Source: CAD feature listing. Evaluate the final solid. Frame: model axes, mm. A direction names the side the tool comes from. Give positions to 0.01 mm unless a question says otherwise; leave off trailing zeros. Loops run counter-clockwise (first coordinate to the right, second up) from the corner with the lowest first, then second, coordinate; pieces in that order, holes last. Notation, with made-up numbers: (37, 87.25) - (65, 87.25) arc R33 cw to (65, 124.25) - close; hole circle Ø3 at (20, 4.25). An arc over 180 degrees is marked (long way). Put each result on its own line as item: value.
```python
from build123d import *

# Parameters (mm, degrees)
SKETCH1_R           = 2
BOSS_EXTRUDE1_DEPTH = 1.6
SKETCH1_3_W         = 8.2
SKETCH1_3_H         = 8.2
SKETCH1_3_W_2       = 6.2
SKETCH1_3_H_2       = 6.2
BOSS_EXTRUDE2_DEPTH = 2
BOSS_EXTRUDE3_START = -0.5
SKETCH1_4_W         = 8.2
SKETCH1_4_H         = 8.2
SKETCH1_4_W_2       = 6.2
SKETCH1_4_H_2       = 6.2
SKETCH1_4_R         = 2
BOSS_EXTRUDE3_DEPTH = 0.5
SKETCH3_W           = 5.8
SKETCH3_H           = 5.8
BOSS_EXTRUDE4_DEPTH = 4.5
CHAMFER1_SIZE       = 0.5
CUT_EXTRUDE1_DEPTH  = 0.2


with BuildPart() as part:
    # Sketch1 → Boss-Extrude1 (new body)
    with BuildSketch(Plane(origin=(0, 0, 0), x_dir=(1, 0, 0), z_dir=(0, 1, 0))):
        with Locations(Location((0, 0, 0), (0, 0, 270))):
            Circle(SKETCH1_R)
    extrude(amount=BOSS_EXTRUDE1_DEPTH)



with BuildPart() as body_2:
    # Sketch1_3 → Boss-Extrude2 (new body)
    with BuildSketch(Plane(origin=(0, 0, 0), x_dir=(1, 0, 0), z_dir=(0, 1, 0))):
        Rectangle(SKETCH1_3_W, SKETCH1_3_H)
        Rectangle(SKETCH1_3_W_2, SKETCH1_3_H_2, mode=Mode.SUBTRACT)
    extrude(amount=BOSS_EXTRUDE2_DEPTH)


with BuildPart() as part_1:
    add(part.part)

    add(body_2.part)  # Boss-Extrude3 merges body 2
    # Sketch1_4 → Boss-Extrude3 (add)
    # profile 1 of 3: a face of its own
    with BuildSketch(Plane(origin=(0, 0, 0), x_dir=(1, 0, 0), z_dir=(0, 1, 0)).offset(BOSS_EXTRUDE3_START)):
        Rectangle(SKETCH1_4_W, SKETCH1_4_H)
        Rectangle(SKETCH1_4_W_2, SKETCH1_4_H_2, mode=Mode.SUBTRACT)
    # profile 2 of 3: a face of its own
    with BuildSketch(Plane(origin=(0, 0, 0), x_dir=(1, 0, 0), z_dir=(0, 1, 0)).offset(BOSS_EXTRUDE3_START)):
        Rectangle(SKETCH1_4_W_2, SKETCH1_4_H_2)
        with Locations(Location((0, 0, 0), (0, 0, 270))):
            Circle(SKETCH1_4_R, mode=Mode.SUBTRACT)
    # profile 3 of 3: a face of its own
    with BuildSketch(Plane(origin=(0, 0, 0), x_dir=(1, 0, 0), z_dir=(0, 1, 0)).offset(BOSS_EXTRUDE3_START)):
        with Locations(Location((0, 0, 0), (0, 0, 270))):
            Circle(SKETCH1_4_R)
    extrude(amount=BOSS_EXTRUDE3_DEPTH)

    # Sketch3 → Boss-Extrude4 (add)
    with BuildSketch(Plane.XZ.offset(0.5)):
        Rectangle(SKETCH3_W, SKETCH3_H)
    extrude(amount=BOSS_EXTRUDE4_DEPTH)

    # Chamfer1
    chamfer1_edges = [part_1.edges().sort_by_distance(p)[0] for p in [
        (2.9, -2.75, -2.9),
        (2.9, -2.75, 2.9),
        (-2.9, -2.75, 2.9),
        (-2.9, -2.75, -2.9),
        (-4.1, 0.75, -4.1),
        (4.1, 0.75, -4.1),
        (4.1, 0.75, 4.1),
        (-4.1, 0.75, 4.1),
    ]]
    chamfer(chamfer1_edges, length=CHAMFER1_SIZE)

    # Sketch4 → Cut-Extrude1 (cut)
    with BuildSketch(Plane.XZ.offset(5)):
        with BuildLine():
            Line((-0.810649843, 2.028880102), (-0.127757215, 2.028880102))
            add(Edge.make_bspline(
                [(-0.127757215, 2.028880102), (-0.094328737, 2.028704351), (-0.029536026, 2.028363703), (0.064683416, 2.023080572), (0.152932226, 2.015876902), (0.235235999, 2.00444681), (0.311556701, 1.990655032), (0.382124338, 1.973953216), (0.44671451, 1.953926603), (0.523827247, 1.922080321), (0.611747908, 1.874757153), (0.7069463, 1.804828588), (0.78835054, 1.719296125), (0.858536857, 1.622813469), (0.914337977, 1.516677698), (0.954707274, 1.403418509), (0.980265149, 1.284496767), (0.982893584, 1.202853589), (0.984221952, 1.161592441)],
                knots=[0, 0, 0, 0, 1.001505555, 1.941167018, 2.826882275, 3.653841531, 4.429895133, 5.150066043, 5.825578002, 6.45369114, 7.647487171, 8.808567382, 9.977351308, 11.170798116, 12.373658725, 13.556498008, 14.765093433, 16, 16, 16, 16], degree=3))
            add(Edge.make_bspline(
                [(0.984221952, 1.161592441), (0.983128733, 1.122939886), (0.980980456, 1.046983969), (0.960437697, 0.935889859), (0.928277028, 0.830138641), (0.883571779, 0.730116255), (0.825469783, 0.638082642), (0.756611464, 0.553295376), (0.673534662, 0.479344319), (0.611291422, 0.438001416), (0.579674676, 0.417001095)],
                knots=[0, 0, 0, 0, 1.044552857, 2.05264487, 3.044412934, 4.028983338, 5.005914585, 5.980388656, 6.974128949, 8, 8, 8, 8], degree=3))
            add(Edge.make_bspline(
                [(0.579674676, 0.417001095), (0.619435104, 0.401736096), (0.695506651, 0.372530372), (0.800192664, 0.320894908), (0.890387509, 0.264732798), (0.966784655, 0.203400947), (1.03212231, 0.137292137), (1.089175251, 0.065437022), (1.137856625, -0.013101736), (1.179569549, -0.097505271), (1.212118305, -0.186911739), (1.236494209, -0.280482515), (1.250461658, -0.377882071), (1.2524493, -0.44416745), (1.253452721, -0.477630315)],
                knots=[0, 0, 0, 0, 1.27268992, 2.434971085, 3.483601985, 4.442670788, 5.356604649, 6.2567628, 7.179492994, 8.113709626, 9.066344395, 10.018646069, 10.999752585, 12, 12, 12, 12], degree=3))
            add(Edge.make_bspline(
                [(1.253452721, -0.477630315), (1.252475875, -0.511797187), (1.250553903, -0.579021465), (1.236373931, -0.6777766), (1.212364824, -0.772151546), (1.179293678, -0.862756729), (1.136131363, -0.949416864), (1.083603399, -1.032230128), (1.020971835, -1.110364458), (0.950908966, -1.184688081), (0.871646821, -1.251515869), (0.786131066, -1.311031575), (0.693284746, -1.359977637), (0.594632752, -1.401093659), (0.489068436, -1.432500857), (0.377065829, -1.454473431), (0.258721527, -1.469278468), (0.177511776, -1.470495673), (0.13586458, -1.471119898)],
                knots=[0, 0, 0, 0, 0.978564426, 1.925352924, 2.850884081, 3.763762016, 4.682927383, 5.618979971, 6.567305752, 7.547517671, 8.540179244, 9.531824382, 10.526200242, 11.540722885, 12.589160233, 13.674978461, 14.80764778, 16, 16, 16, 16], degree=3))
            Line((0.13586458, -1.471119898), (-0.810649843, -1.471119898))
            Line((-0.810649843, -1.471119898), (-0.810649843, 2.028880102))
        make_face()
        with BuildLine():
            Line((-0.496547279, 1.669905743), (-0.496547279, 0.548110871))
            Line((-0.496547279, 0.548110871), (-0.285509619, 0.548110871))
            add(Edge.make_bspline(
                [(-0.285509619, 0.548110871), (-0.254660823, 0.548510794), (-0.195054664, 0.549283527), (-0.108734767, 0.551497044), (-0.028609749, 0.557695087), (0.045182084, 0.563891349), (0.112524528, 0.573965937), (0.173268389, 0.58595806), (0.228366986, 0.598640965), (0.291906532, 0.620210452), (0.36397948, 0.652088127), (0.440812584, 0.701559963), (0.508547054, 0.760484316), (0.565744242, 0.828475278), (0.612555712, 0.903341464), (0.645069427, 0.983888344), (0.667116712, 1.068108476), (0.669108243, 1.125926729), (0.670119388, 1.155282345)],
                knots=[0, 0, 0, 0, 1.156816544, 2.235205308, 3.236616184, 4.169592532, 5.011045266, 5.787822928, 6.49130361, 7.128639758, 8.301311294, 9.436451833, 10.541879658, 11.654887649, 12.756523258, 13.837046038, 14.901820046, 16, 16, 16, 16], degree=3))
            add(Edge.make_bspline(
                [(0.670119388, 1.155282345), (0.669593208, 1.174708117), (0.668561048, 1.212813889), (0.660107745, 1.268363243), (0.645740171, 1.320606996), (0.627285877, 1.370261106), (0.601497189, 1.415772956), (0.571133725, 1.458716152), (0.534448035, 1.49762827), (0.492690722, 1.533997769), (0.4446821, 1.566242296), (0.390450808, 1.59448306), (0.329263131, 1.617223836), (0.262150276, 1.637139989), (0.188079188, 1.651128283), (0.107904635, 1.66278167), (0.020969916, 1.668714412), (-0.039175187, 1.669499775), (-0.070265228, 1.669905743)],
                knots=[0, 0, 0, 0, 0.91205012, 1.789085906, 2.630437955, 3.453916878, 4.269457761, 5.079663411, 5.91843418, 6.774407191, 7.675494373, 8.627863946, 9.638891023, 10.736472738, 11.911756761, 13.175263542, 14.539845004, 16, 16, 16, 16], degree=3))
            Line((-0.070265228, 1.669905743), (-0.496547279, 1.669905743))
        make_face(mode=Mode.SUBTRACT)
        with BuildLine():
            Line((-0.496547279, 0.189136512), (-0.496547279, -1.112145539))
            Line((-0.496547279, -1.112145539), (-0.049231574, -1.112145539))
            add(Edge.make_bspline(
                [(-0.049231574, -1.112145539), (-0.017212648, -1.111761792), (0.044499611, -1.111022169), (0.133600841, -1.108607615), (0.216183945, -1.103115339), (0.29187208, -1.09446949), (0.361482533, -1.08509104), (0.424180236, -1.072479759), (0.480473429, -1.058030799), (0.545747737, -1.035696627), (0.619251245, -1.001000156), (0.698462102, -0.948685929), (0.76888832, -0.886362622), (0.828693579, -0.814231707), (0.877706568, -0.73580038), (0.913362023, -0.65265503), (0.93535288, -0.566169503), (0.938015049, -0.507202791), (0.939350157, -0.477630315)],
                knots=[0, 0, 0, 0, 1.160039823, 2.235823828, 3.228722157, 4.157150951, 4.99529583, 5.772374946, 6.472645482, 7.099169577, 8.269452708, 9.405989375, 10.527446681, 11.663510218, 12.788923519, 13.866172445, 14.929861265, 16, 16, 16, 16], degree=3))
            add(Edge.make_bspline(
                [(0.939350157, -0.477630315), (0.939074053, -0.459136974), (0.938526298, -0.422448593), (0.930265683, -0.368532773), (0.918251813, -0.3163069), (0.902720379, -0.26562916), (0.880100912, -0.217415783), (0.853694367, -0.170713224), (0.822732965, -0.125459744), (0.774488799, -0.068247491), (0.704316815, -0.002330478), (0.604610039, 0.062207024), (0.491237741, 0.114254831), (0.409010249, 0.136354308), (0.366533651, 0.147770326)],
                knots=[0, 0, 0, 0, 0.723448775, 1.435228256, 2.130040452, 2.821711965, 3.505591119, 4.210454504, 4.921174351, 5.648778258, 7.137944449, 8.670945889, 10.280296675, 12, 12, 12, 12], degree=3))
            add(Edge.make_bspline(
                [(0.366533651, 0.147770326), (0.349504555, 0.15122541), (0.312581962, 0.158716745), (0.252374382, 0.166624448), (0.183638513, 0.173669508), (0.106215636, 0.178880666), (0.020007795, 0.184267209), (-0.075169124, 0.18636203), (-0.178926439, 0.18886129), (-0.250918811, 0.189042425), (-0.288314106, 0.189136512)],
                knots=[0, 0, 0, 0, 0.634451884, 1.375622551, 2.216452059, 3.157844607, 4.20941857, 5.370758133, 6.634282058, 8, 8, 8, 8], degree=3))
            Line((-0.288314106, 0.189136512), (-0.496547279, 0.189136512))
        make_face(mode=Mode.SUBTRACT)
    extrude(amount=-CUT_EXTRUDE1_DEPTH, mode=Mode.SUBTRACT)


solid = part_1.part
```
1) Section query B-B, the plane z = 2.25. Output: boundary loops of the cut face in (x, y), plus the area to 3 significant figures.
Check result:
outline: (-4.1, -0.5) - (-2.9, -0.5) - (-2.9, -5) - (2.9, -5) - (2.9, -0.5) - (4.1, -0.5) - (4.1, 2) - (3.1, 2) - (3.1, 0) - (-3.1, 0) - (-3.1, 2) - (-4.1, 2) - close
area: 34.2 mm²
2) Section query C-C, the plane y = -3.25. Output: boundary loops of the cut face in (x, z), plus the area to 3 significant figures.
Check result:
outline: (-2.9, -2.4) - (-2.4, -2.9) - (2.4, -2.9) - (2.9, -2.4) - (2.9, 2.4) - (2.4, 2.9) - (-2.4, 2.9) - (-2.9, 2.4) - close
area: 33.1 mm²
3) Section query D-D, the plane x = -1.25. Output: boundary loops of the cut face in (y, z).
Check result:
outline: (-5, -2.9) - (-0.5, -2.9) - (-0.5, -4.1) - (2, -4.1) - (2, -3.1) - (0, -3.1) - (0, -1.56) - (1.6, -1.56) - (1.6, 1.56) - (0, 1.56) - (0, 3.1) - (2, 3.1) - (2, 4.1) - (-0.5, 4.1) - (-0.5, 2.9) - (-5, 2.9) - close
4) Pin query (flat end, axial travel): P1, Ø1, axis at y = -2, z = -2.5, coming from the +X side; P2, Ø3, axis at x = 3, y = -3.5, coming from the +Z side; P3, Ø1, axis at y = -2.5, z = -2.5, coming from the -X side; P4, Ø2, axis at x = -2.5, z = 0.5, coming from the +Y side. Return the tip coordinate at first contact, or that it passes through.
Check result:
P1: x = 2.9
P2: z = 2.9
P3: x = -2.9
P4: y = 2
5) Section query A-A, the plane y = 1. Output: boundary loops of the cut face in (x, z), plus the area to 3 significant figures.
Check result:
outline: (-4.1, -3.6) - (-3.6, -4.1) - (3.6, -4.1) - (4.1, -3.6) - (4.1, 3.6) - (3.6, 4.1) - (-3.6, 4.1) - (-4.1, 3.6) - close; circle Ø4 at (0, 0); hole (-3.1, -3.1) - (3.1, -3.1) - (3.1, 3.1) - (-3.1, 3.1) - close
area: 40.9 mm²
6) Mould query, pull axis X, two halves, no side actions, for faces 1 (the flat face through (0, 1, -4.1)), 2 (the flat face through (-1, 0, -2)), 3 (the flat face through (4.1, 1, 0)). Classes: pulls with the +X half, pulls with the -X half, needs draft (parallel to the pull), parting line crosses it, or undercut.
Check result:
face 1: needs draft
face 2: undercut
face 3: pulls with the +X half
7) Access query for faces 4 (the flat face through (0, -3, 2.9)), 5 (the flat face through (2.9, -3, 0)), 6 (the flat face through (0.47, -4.8, 0.3)), 7 (the flat face through (0, -3, -2.9)). Directions: +Z, -Z, +X, -X, +Y, -Y. A direction counts if a zero-diameter tool reaches every point of the face in a straight line with its end or side. Return the directions, or none.
Check result:
face 4: +Z, +X, -X, -Y
face 5: +Z, -Z, +X, -Y
face 6: -Y
face 7: -Z, +X, -X, -Y
8) Material intervals for line 1 along X through (y, z) = (0.5, -0.25); line 2 along X through (y, z) = (1.5, 3); line 3 along Z through (x, y) = (1, -3), sorted ascending. Write a range as [from, to].
Check result:
line 1: [-4.1, -3.1], [-1.98, 1.98], [3.1, 4.1]
line 2: [-4.1, -3.1], [3.1, 4.1]
line 3: [-2.9, 2.9]
